```python
from build123d import *

# Parameters (mm, degrees)
SKETCH_1_W          = 26
SKETCH_1_H          = 18
EXTRUDE_1_DEPTH     = 4
SKETCH_2_W          = 0.9
SKETCH_2_H          = 6
CUT_EXTRUDE_1_DEPTH = 27
SKETCH_3_R          = 1.5
CUT_EXTRUDE_2_DEPTH = 4


with BuildPart() as part:
    # 草图1 → 凸台-拉伸1 (new body)
    with BuildSketch(Plane.XY):
        with Locations((13, 9)):
            Rectangle(SKETCH_1_W, SKETCH_1_H)
    extrude(amount=EXTRUDE_1_DEPTH)

    # 草图2 → 切除-拉伸1 (cut, through all)
    with BuildSketch(Plane(origin=(26, 0, 0), x_dir=(0, 0, -1), z_dir=(1, 0, 0))):
        with Locations((-3.55, 3)):
            Rectangle(SKETCH_2_W, SKETCH_2_H)
        with Locations((-3.55, 15)):
            Rectangle(SKETCH_2_W, SKETCH_2_H)
    extrude(amount=-CUT_EXTRUDE_1_DEPTH, mode=Mode.SUBTRACT)

    # 草图3 → 切除-拉伸2 (cut)
    with BuildSketch(Plane.XY.offset(3.1)):
        with Locations((5.5, 14.5)):
            Circle(SKETCH_3_R)
        with Locations((5.5, 3.5)):
            Circle(SKETCH_3_R)
        with Locations((20.5, 3.5)):
            Circle(SKETCH_3_R)
        with Locations((20.5, 14.5)):
            Circle(SKETCH_3_R)
    extrude(amount=-CUT_EXTRUDE_2_DEPTH, mode=Mode.SUBTRACT)


solid = part.part
```
The listing builds one solid part. Answer for the finished solid, in the listing's coordinates (mm). A direction names the side the tool comes from. Give positions to 0.01 mm unless a question says otherwise; leave off trailing zeros. Order: outer loops, then holes, each group sorted by start corner. A loop starts at its lowest first (then second) coordinate and runs counter-clockwise, first axis right, second up. Notation, with made-up numbers: M 21.25,73.25 L 36.25,73.25 A10 cw 36.25,83.25 Z; hole C 70,41 d3. An arc over 180 degrees is marked long. Put each result on its own line as item: value. Start each with the question number.
Item 1: Which of the six approach directions +Z, -Z, +X, -X, +Y, -Y give full straight-line access (tool end or side, diameter ignored) to faces 4 (the face through (13, 15, 3.1)), 5 (the face through (13.2, 6, 3.6)), 6 (the face through (13, 18, 2))?
Item 2: Flat-ended cylindrical pins translate along their axes: P1, Ø4, axis at x = 5.5, y = 3.5, coming from the -Z side; P2, Ø2.5, axis at x = 5.5, y = 14.5, coming from the -Z side; P3, Ø0.7, axis at x = 6.5, z = 3.5, coming from the +Y side; P4, Ø3.5, axis at x = 20.5, y = 14.5, coming from the +Z side. Find the tip coordinate at first contact, or state that the pin passes through.
Item 3: The part is cut by section B-B, the plane x = 20.5. Determine the outline of the cut face in (y, z), and give its area (3 significant figures).
Item 4: Find the intervals of material crossed by line 1 along Y through (x, z) = (20.5, 0.8); line 2 along X through (y, z) = (13.5, 0.9); line 3 along Y through (x, z) = (4.5, 2.05), in increasing order.
Item 5: The part is cut by section D-D, the plane z = 0.8. Determine the outline of the cut face in (x, y), and give its area (3 significant figures).
Item 6: The part is cut by section C-C, the plane x = 2. Determine the outline of the cut face in (y, z), and give its area (3 significant figures).
Item 7: The part is cut by section A-A, the plane y = 3.5. Determine the outline of the cut face in (x, z), and give its area (3 significant figures).
Item 8: For a pull along Y with two mould halves and no side action, classify faces 1 (the face through (13.2, 12, 3.6)), 2 (the face through (13, 9, 0)), 3 (the face through (19, 14.57, 1.57)) as +Y half, -Y half, draft (parallel to the pull), parting line (faces both ways), or undercut.
Answer key:
1. face 4: +Z, +X, -X, +Y
1. face 5: +Z, +X, -X, -Y
1. face 6: +Z, -Z, +X, -X, +Y
2. P1: stops at z = 0
2. P2: passes through
2. P3: stops at y = 12
2. P4: stops at z = 3.1
3. outline: M 0,0 L 2,0 L 2,3.1 L 0,3.1 Z; M 5,0 L 13,0 L 13,3.1 L 12,3.1 L 12,4 L 6,4 L 6,3.1 L 5,3.1 Z; M 16,0 L 18,0 L 18,3.1 L 16,3.1 Z
3. area: 42.6 mm²
4. line 1: y = 0 to 2, 5 to 13, 16 to 18
4. line 2: x = 0 to 4.38, 6.62 to 19.38, 21.62 to 26
4. line 3: y = 0 to 2.38, 4.62 to 13.38, 15.62 to 18
5. outline: M 0,0 L 26,0 L 26,18 L 0,18 Z; hole C 5.5,3.5 d3; hole C 5.5,14.5 d3; hole C 20.5,3.5 d3; hole C 20.5,14.5 d3
5. area: 440 mm²
6. outline: M 0,0 L 18,0 L 18,3.1 L 12,3.1 L 12,4 L 6,4 L 6,3.1 L 0,3.1 Z
6. area: 61.2 mm²
7. outline: M 0,0 L 4,0 L 4,3.1 L 0,3.1 Z; M 7,0 L 19,0 L 19,3.1 L 7,3.1 Z; M 22,0 L 26,0 L 26,3.1 L 22,3.1 Z
7. area: 62.0 mm²
8. face 1: +Y half
8. face 2: draft
8. face 3: undercut
